Read the model definition and answer for the solid it produces. Units are mm, in the model's axes. Face numbers are marked on the shaded views. A direction names the side the tool comes from. Coordinates: 2 decimals unless noted, no trailing zeros. Write each loop counter-clockwise with the first axis right and the second up, starting at its lowest first coordinate (ties: lowest second). Pieces come first, ordered by that corner, then holes.
(1) Determine the mould class of the marked faces 1 and 2 for opening direction X: pulls with the +X half, pulls with the -X half, needs draft (parallel to the pull), parting line crosses it, or undercut.
(2) Which of the six approach directions +Z, -Z, +X, -X, +Y, -Y give full straight-line access (tool end or side, diameter ignored) to the marked faces 3 and 4?
(3) Given pin 1 (2 mm diameter, centred on x = -6, z = 6.5, fed in from -Y); pin 2 (5 mm diameter, centred on x = -7, y = 6, fed in from -Z); pin 3 (1 mm diameter, centred on x = -4, y = 3, fed in from -Z), each flat-ended and moving along its own axis, determine where each tip first touches the part or whether it passes through.
(4) Straight lines are drawn through the part: line 1 along Y through (x, z) = (-6.25, 1.25); line 2 along X through (y, z) = (2, 0); line 3 along X through (y, z) = (3.25, 1). For each, find the intervals that lie inside material, in ascending order.
(5) The part is cut by section A-A, the plane z = -4.75. Determine the outline of the cut face in (x, y), and give its area (3 significant figures).
```python
from build123d import *

# Parameters (mm, degrees)
BOSS_EXTRUDE1_REACH = 17.033
CIRPATTERN1_COUNT   = 20
SKETCH3_R           = 7.5
SKETCH3_R_2         = 6.75
CUT_EXTRUDE1_DEPTH  = 7


with BuildPart() as part:
    # Sketch1 → Revolve1 (revolve)
    with BuildSketch(Plane.XY, mode=Mode.PRIVATE) as revolve1_sk:
        Polygon((-2.5, 0), (-9, 0), (-9, 1), (-6.05, 1), (-6.05, 8), (-9, 8), (-9, 9), (-2.5, 9), align=None)
    revolve(revolve1_sk.sketch.rotate(Axis((0, 0, 0), (0, 1, 0)), 270), axis=Axis((0, 0, 0), (0, 1, 0)))

    # Sketch2 → Boss-Extrude1 (add, up to next)
    with BuildSketch(Plane(origin=(0, 1, 0), x_dir=(1, 0, 0), z_dir=(0, 1, 0)), mode=Mode.PRIVATE) as boss_extrude1_sk1:
        Polygon((-6.946844773, 0), (-5.946844773, -1), (-5.946844773, 1), align=None)
    boss_extrude1_tool1 = extrude(boss_extrude1_sk1.sketch, amount=BOSS_EXTRUDE1_REACH, mode=Mode.PRIVATE) - part.part
    boss_extrude1 = boss_extrude1_tool1.solids().sort_by_distance((-6.280178, 1, 0))[0]
    add(boss_extrude1)

    # CirPattern1: Boss-Extrude1 ×20 about axis
    cirpattern1_axis = Axis((0, 0, 0), (0, 1, 0))
    for i in range(1, CIRPATTERN1_COUNT):
        add(boss_extrude1.rotate(cirpattern1_axis, i * 360 / CIRPATTERN1_COUNT))

    # Sketch3 → Cut-Extrude1 (cut)
    with BuildSketch(Plane(origin=(0, 1, 0), x_dir=(1, 0, 0), z_dir=(0, 1, 0))):
        Circle(SKETCH3_R)
        Circle(SKETCH3_R_2, mode=Mode.SUBTRACT)
    extrude(amount=CUT_EXTRUDE1_DEPTH, mode=Mode.SUBTRACT)


solid = part.part
```
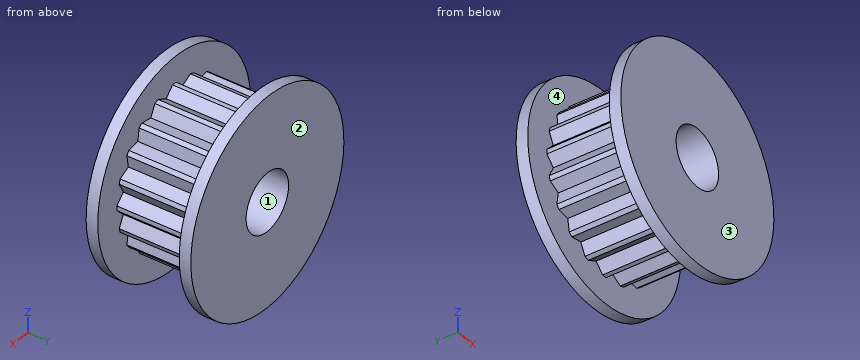
Computed:
1. face 1: undercut
1. face 2: needs draft
2. face 3: +Z, -Z, +X, -X, -Y
2. face 4: none
3. pin 1: stops at y = 0
3. pin 2: stops at z = -7.12
3. pin 3: stops at z = -5.58
4. line 1: y = 0 to 1, 8 to 9
4. line 2: x = -6.75 to -2.5, 2.5 to 6.75
4. line 3: x = -6.02 to -2.29, 2.29 to 6.02
5. outline: (-7.64, 0) - (7.64, 0) - (7.64, 1) - (4.22, 1) - (4.22, 8) - (7.64, 8) - (7.64, 9) - (-7.64, 9) - (-7.64, 8) - (-4.22, 8) - (-4.22, 1) - (-7.64, 1) - close
5. area: 89.7 mm2
